Drawing for the job (mm, zero at the part's lowest x, y, z). A direction names the side the tool comes from. Coordinates: 2 decimals unless noted, no trailing zeros. Order: outer loops, then holes, each group sorted by start corner. A loop starts at its lowest first (then second) coordinate and runs counter-clockwise, first axis right, second up.
1) Pin check, flat tip, straight feed: pin 1 Ø2 at (x, z) = (3.46, 3) entering from -Y. Stop position of the tip, or through.
2) Cut at D-D (z = 4). List the corners of the cut face in (x, y).
3) Cut at A-A (y = 1.25). List the corners of the cut face in (x, z).
4) Cut at C-C (y = 7.25). List the corners of the cut face in (x, z), and give its area (3 significant figures).
5) Cut at B-B (x = 4). List the corners of the cut face in (y, z), and give its area (3 significant figures).
6) Tool access for the marked faces 4 and 5: list every direction of +Z, -Z, +X, -X, +Y, -Y with a clear straight run to the whole face (end or side of a thin tool).
7) Wall check: L1, parallel to Y at x = 0.75, z = 3.5; L2, parallel to Z at x = 2.5, y = 4; L3, parallel to Y at x = 2.25, z = 2.9. Give the ranges that are in metal, low to high.
8) Mould opens along Z. For the marked faces 1, 2 and 3 say: +Z half, -Z half, draft (parallel to the pull), parting line (faces both ways), or undercut.
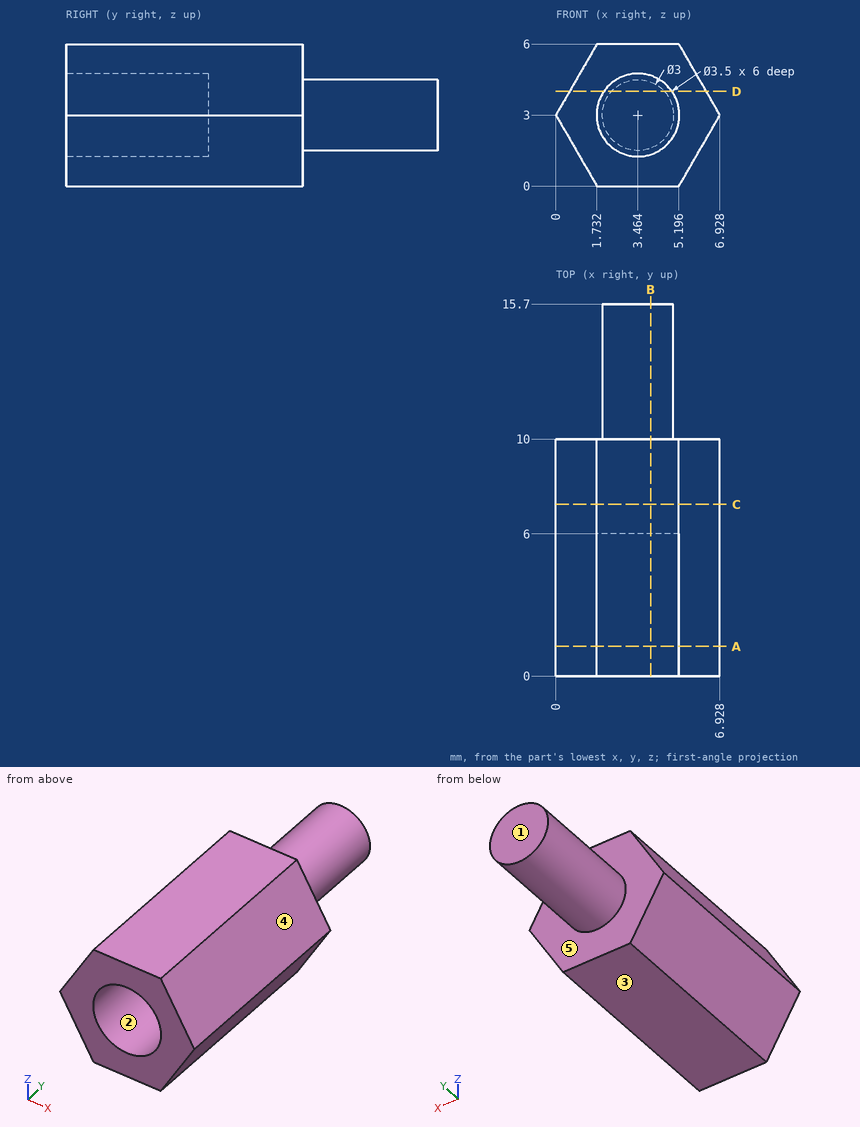
Geometry check:
1. pin 1: stops at y = 6
2. outline: (0.58, 0) - (2.03, 0) - (2.03, 6) - (4.9, 6) - (4.9, 0) - (6.35, 0) - (6.35, 10) - (4.58, 10) - (4.58, 15.7) - (2.35, 15.7) - (2.35, 10) - (0.58, 10) - close
3. outline: (0, 3) - (1.73, 0) - (5.2, 0) - (6.93, 3) - (5.2, 6) - (1.73, 6) - close; hole circle Ø3.5 at (3.46, 3)
4. outline: (0, 3) - (1.73, 0) - (5.2, 0) - (6.93, 3) - (5.2, 6) - (1.73, 6) - close
4. area: 31.2 mm2
5. outline: (0, 0) - (10, 0) - (10, 1.6) - (15.7, 1.6) - (15.7, 4.4) - (10, 4.4) - (10, 6) - (0, 6) - (0, 4.67) - (6, 4.67) - (6, 1.33) - (0, 1.33) - close
5. area: 56.0 mm2
6. face 4: +Z, +X, +Y, -Y
6. face 5: +Y
7. L1: y = 0 to 10
7. L2: z = 0 to 1.54, 4.46 to 6
7. L3: y = 6 to 15.7
8. face 1: draft
8. face 2: undercut
8. face 3: -Z half
